from build123d import *

# Parameters (mm, degrees)
BOSS_EXTRUDE1_DEPTH = 1934
FILLET1_R           = 3
SKETCH2_W           = 90
SKETCH2_H           = 30
CUT_EXTRUDE1_DEPTH  = 6
SKETCH3_W           = 90
SKETCH3_H           = 30
CUT_EXTRUDE2_DEPTH  = 6


with BuildPart() as part:
    # Sketch1 → Boss-Extrude1 (new body)
    with BuildSketch(Plane(origin=(0, 0, 0), x_dir=(0, 0, -1), z_dir=(1, 0, 0))):
        Polygon((0, 0), (25, 0), (25, 47), (-13, 47), (-13, 77), (-10, 77), (-10, 50), (28, 50), (28, -3), (0, -3), align=None)
    extrude(amount=BOSS_EXTRUDE1_DEPTH)

    # Fillet1
    fillet1_edges = [part.edges().sort_by_distance(p)[0] for p in [
        (967, 0, -25),
        (967, 47, -25),
        (967, 47, 13),
        (967, 50, 10),
        (967, 50, -28),
        (967, -3, -28),
    ]]
    fillet(fillet1_edges, radius=FILLET1_R)

    # Sketch2 → Cut-Extrude1 (cut)
    with BuildSketch(Plane.XY.offset(13)):
        with Locations((45, 62)):
            Rectangle(SKETCH2_W, SKETCH2_H)
    extrude(amount=-CUT_EXTRUDE1_DEPTH, mode=Mode.SUBTRACT)

    # Sketch3 → Cut-Extrude2 (cut)
    with BuildSketch(Plane.XY.offset(13)):
        with Locations((1889, 62)):
            Rectangle(SKETCH3_W, SKETCH3_H)
    extrude(amount=-CUT_EXTRUDE2_DEPTH, mode=Mode.SUBTRACT)


solid = part.part
Source: CAD feature listing. Evaluate the final solid. Frame: model axes, mm. A direction names the side the tool comes from. Give positions to 0.01 mm unless a question says otherwise; leave off trailing zeros. Loops run counter-clockwise (first coordinate to the right, second up) from the corner with the lowest first, then second, coordinate; pieces in that order, holes last. Notation, with made-up numbers: (-25.5, -3) -> (-15.5, -3) arc R27 cw to (-15.5, 26) -> close; hole circle Ø7 at (87.5, 4.5). An arc over 180 degrees is marked (long way). Use a Markdown table: item, result. Add a question column.
1) Line query: line 1 along Y through (x, z) = (1333, -10.5); line 2 along Z through (x, y) = (1279.5, 58); line 3 along Y through (x, z) = (850, 5). Output: solid intervals per line, ascending. Write a range as [from, to].
2) First-contact query: pin 1 (5 mm diameter, centred on x = 1194, z = 3, fed in from -Y); pin 2 (3.5 mm diameter, centred on x = 1906, y = 48, fed in from +Z); pin 3 (3 mm diameter, centred on y = 69, z = 9.5, fed in from +X). Flat tips, straight axial feed; report the tip coordinate or a pass-through.
3) Reachability of faces 1 (the face through (953, 47, -6)), 2 (the face through (0, 28, -26)) from +Z, -Z, +X, -X, +Y, -Y: full face, straight path, thin tool, end or side. Return the list, or none.
4) Section query B-B, the plane z = -13. Return the cut outline in (x, y), then the cut area to 3 significant figures.
5) Section query C-C, the plane y = 23.5. Return the cut outline in (x, z).
6) Section query A-A, the plane x = 1526.5. Return the cut outline in (y, z).
7) Pull-direction query (Y, two-part tool) for faces 3 (the face through (953, 50, -9)), 4 (the face through (953, 23, -25)), 5 (the face through (953, 24, -28)); classes: +Y half, -Y half, draft (parallel to the pull), parting line (faces both ways), or undercut.
Numbers:
| question | item | result |
|---|---|---|
| 1 | line 1 | y = [-3, 0], [47, 50] |
| 1 | line 2 | z = [10, 13] |
| 1 | line 3 | y = [47, 50] |
| 2 | pin 1 | stops at y = 47 |
| 2 | pin 2 | stops at z = 7 |
| 2 | pin 3 | stops at x = 1844 |
| 3 | face 1 | +Z, +X, -X |
| 3 | face 2 | +Z, -Z, -X, +Y, -Y |
| 4 | outline | (0, -3) -> (1934, -3) -> (1934, 0) -> (0, 0) -> close; (0, 47) -> (1934, 47) -> (1934, 50) -> (0, 50) -> close |
| 4 | area | 11,600 mm2 |
| 5 | outline | (0, -28) -> (1934, -28) -> (1934, -25) -> (0, -25) -> close |
| 6 | outline | (-3, -25) arc R3 ccw to (0, -28) -> (47, -28) arc R3 ccw to (50, -25) -> (50, 7) arc R3 cw to (53, 10) -> (77, 10) -> (77, 13) -> (50, 13) arc R3 ccw to (47, 10) -> (47, -22) arc R3 cw to (44, -25) -> (3, -25) arc R3 cw to (0, -22) -> (0, 0) -> (-3, 0) -> close |
| 7 | face 3 | +Y half |
| 7 | face 4 | undercut |
| 7 | face 5 | draft |
